from build123d import *

# Parameters (mm, degrees)
SKETCH1_W           = 3.95
SKETCH1_H           = 50.3
BOSS_EXTRUDE1_DEPTH = 1.25
SKETCH4_W           = 6.5
SKETCH4_H           = 3
BOSS_EXTRUDE2_DEPTH = 1.25
SKETCH5_OUTSIDE_W   = 26.39
SKETCH5_OUTSIDE_H   = 26.39
SKETCH5_OUTSIDE_R   = 6.5
CUT_EXTRUDE1_DEPTH  = 54.9


with BuildPart() as part:
    # Sketch1 → Revolve1 (revolve)
    with BuildSketch(Plane.XY):
        with Locations((1.975, -25.15)):
            Rectangle(SKETCH1_W, SKETCH1_H)
    revolve(axis=Axis((0, 6.295, 0), (0, -1, 0)))

    # Sketch2 → Revolve2 (revolve)
    with BuildSketch(Plane.XY):
        Polygon((0, 0), (6.5, 0), (6.5, 2.5), (5, 3.6), (3.5, 3.6), (3.5, 2.7), (0, 2.7), align=None)
    revolve(axis=Axis((0, 6.295, 0), (0, -1, 0)))

    # Sketch3 → Boss-Extrude1 (add)
    with BuildSketch(Plane(origin=(0, 0, 0), x_dir=(0.766044443, 0, -0.64278761), z_dir=(0.64278761, 0, 0.766044443))):
        Polygon((0, 0), (6.5, 0), (0, -6.5), align=None)
    extrude(amount=-BOSS_EXTRUDE1_DEPTH)

    # Sketch4 → Boss-Extrude2 (add)
    with BuildSketch(Plane(origin=(0, 0, 0), x_dir=(0.766044443, 0, -0.64278761), z_dir=(0.64278761, 0, 0.766044443))):
        with Locations((3.25, -1.5)):
            Rectangle(SKETCH4_W, SKETCH4_H)
    extrude(amount=BOSS_EXTRUDE2_DEPTH)

    # Sketch5 outside → Cut-Extrude1 (cut, through all)
    with BuildSketch(Plane(origin=(0, 3.6, 0), x_dir=(1, 0, 0), z_dir=(0, 1, 0))):
        Rectangle(SKETCH5_OUTSIDE_W, SKETCH5_OUTSIDE_H)
        Circle(SKETCH5_OUTSIDE_R, mode=Mode.SUBTRACT)
    extrude(amount=-CUT_EXTRUDE1_DEPTH, mode=Mode.SUBTRACT)


solid = part.part
The model under review builds one solid part; all positions refer to its coordinate system, in mm. A direction names the side the tool comes from. Give positions to 0.01 mm unless a question says otherwise; leave off trailing zeros. Order: outer loops, then holes, each group sorted by start corner. A loop starts at its lowest first (then second) coordinate and runs counter-clockwise, first axis right, second up. Notation, with made-up numbers: M 30,-7.5 L 82,-7.5 A26 cw 82,23.5 Z; hole C -29,83 d2. An arc over 180 degrees is marked long. Answer in a Markdown table with one row per item. Add a question column.
1. Mouldability with a two-part tool opening along Z and no side actions: class faces 4 (the cylindrical face through (6.2, 1.01, -1.95)), 5 (the cylindrical face through (3.233, 3.144, -1.341)), 6 (the flat face through (2.2, 3.6, -3.3)) as released by +Z, released by -Z, zero draft, split by the parting line, or undercut.
2. Add section B-B on x = 0. State the section outline as (y, z) points.
3. For pin 1 Ø1.5 at (y, z) = (-44.5, 1.5) entering from -X; pin 2 Ø6.5 at (x, z) = (0, 0) entering from +Y; pin 3 Ø5 at (x, y) = (-0.5, -5.5) entering from -Z; pin 4 Ø1 at (x, z) = (3, 0.5) entering from +Y, all flat-tipped, find the tip position at first contact; note any pin that passes through.
4. Add section A-A on z = 0. State the section outline as (x, y) points, plus the area to 3 significant figures.
5. To check wall thickness, follow line 1 along Z through (x, y) = (0, 3.25); line 2 along Z through (x, y) = (0.25, -5.5); line 3 along Y through (x, z) = (-4.5, -2). State the ranges of each line that lie inside material, in increasing order.
6. Machinability: for faces 1 (the flat face through (-3, 0, -3)), 2 (the flat face through (4, -3, -3)), 3 (the flat face through (2.865, -1.051, -4.036)), which of the approach directions +Z, -Z, +X, -X, +Y, -Y give a long, thin tool a straight path to every point of the face, cutting with its end or side? Answer none if there is none.
7. Add section C-C on y = -20. State the section outline as (x, z) points, plus the area to 3 significant figures.
The answers:
| question | item | result |
|---|---|---|
| 1 | face 4 | split by the parting line |
| 1 | face 5 | undercut |
| 1 | face 6 | zero draft |
| 2 | outline | M -50.3,-3.95 L 0,-3.95 L 0,-6.5 L 2.5,-6.5 L 3.6,-5 L 3.6,-3.5 L 2.7,-3.5 L 2.7,3.5 L 3.6,3.5 L 3.6,5 L 2.5,6.5 L 0,6.5 L 0,3.95 L -50.3,3.95 Z |
| 3 | pin 1 | x = -3.88 |
| 3 | pin 2 | y = 2.7 |
| 3 | pin 3 | z = -3.95 |
| 3 | pin 4 | y = 3.6 |
| 4 | outline | M -6.5,0 L -3.95,0 L -3.95,-50.3 L 3.95,-50.3 L 3.95,0 L 6.5,0 L 6.5,2.5 L 5,3.6 L 3.5,3.6 L 3.5,2.7 L -3.5,2.7 L -3.5,3.6 L -5,3.6 L -6.5,2.5 Z |
| 4 | area | 436 mm2 |
| 5 | line 1 | -5.48 to -3.5, 3.5 to 5.48 |
| 5 | line 2 | -3.94 to 3.94 |
| 5 | line 3 | 0 to 3.6 |
| 6 | face 1 | -Y |
| 6 | face 2 | -Z, +X, -Y |
| 6 | face 3 | -Z, -Y |
| 7 | outline | C 0,0 d7.9 |
| 7 | area | 49.0 mm2 |
